from build123d import *

# Parameters (mm, degrees)
SKETCH1_R            = 11
SKETCH1_R_2          = 3
BOSS_EXTRUDE2_DEPTH  = 6
SKETCH3_R            = 10.5
CUT_EXTRUDE1_DEPTH   = 1
SKETCH4_R            = 3.55
BOSS_EXTRUDE5_DEPTH  = 1
SKETCH5_R            = 3.05
CUT_EXTRUDE2_DEPTH   = 17.673332001
BOSS_EXTRUDE6_START  = 2
SKETCH6_R            = 3.55
BOSS_EXTRUDE6_DEPTH  = 2
SKETCH7_R            = 3.05
CUT_EXTRUDE3_DEPTH   = 18.492855685
SKETCH9_R            = 11
BOSS_EXTRUDE9_DEPTH  = 6
SKETCH10_W           = 46.121208306
SKETCH10_H           = 4.65
BOSS_EXTRUDE10_DEPTH = 6


with BuildPart() as part:
    # Sketch1 → Boss-Extrude2 (new body)
    with BuildSketch(Plane.XY):
        Circle(SKETCH1_R)
        Circle(SKETCH1_R_2, mode=Mode.SUBTRACT)
    extrude(amount=BOSS_EXTRUDE2_DEPTH)

    # Sketch3 → Cut-Extrude1 (cut)
    with BuildSketch(Plane.XY.offset(6)):
        Circle(SKETCH3_R)
    extrude(amount=-CUT_EXTRUDE1_DEPTH, mode=Mode.SUBTRACT)

    # Sketch4 → Boss-Extrude5 (add)
    with BuildSketch(Plane.XY.offset(5)):
        Circle(SKETCH4_R)
    extrude(amount=BOSS_EXTRUDE5_DEPTH)

    # Sketch5 → Cut-Extrude2 (cut, through all)
    with BuildSketch(Plane.XY.offset(6)):
        Circle(SKETCH5_R)
    extrude(amount=-CUT_EXTRUDE2_DEPTH, mode=Mode.SUBTRACT)

    # Sketch6 → Boss-Extrude6 (add)
    with BuildSketch(Plane(origin=(0, 0, 0), x_dir=(-1, 0, 0), z_dir=(0, 0, -1)).offset(BOSS_EXTRUDE6_START)):
        with Locations(Location((0, 0, 0), (0, 0, 180))):
            Circle(SKETCH6_R)
    extrude(amount=-BOSS_EXTRUDE6_DEPTH)

    # Sketch7 → Cut-Extrude3 (cut, through all)
    with BuildSketch(Plane(origin=(0, 0, -2), x_dir=(-1, 0, 0), z_dir=(0, 0, -1))):
        with Locations(Location((0, 0, 0), (0, 0, 180))):
            Circle(SKETCH7_R)
    extrude(amount=-CUT_EXTRUDE3_DEPTH, mode=Mode.SUBTRACT)

    # Sketch9 → Boss-Extrude9 (add, through all)
    with BuildSketch(Plane.XY):
        with BuildLine():
            Line((-12.660604153, 0), (-12.660604153, -9.354915786))
            Line((-12.660604153, -9.354915786), (-23.060604153, -9.354915786))
            Line((-23.060604153, -9.354915786), (-23.060604153, -15.354915786))
            Line((-23.060604153, -15.354915786), (23.060604153, -15.354915786))
            Line((23.060604153, -15.354915786), (23.060604153, -9.354915786))
            Line((23.060604153, -9.354915786), (12.660604153, -9.354915786))
            Line((12.660604153, -9.354915786), (12.660604153, 0))
            ThreePointArc((12.660604153, 0), (0, 12.660604153), (-12.660604153, 0))
        make_face()
        Circle(SKETCH9_R, mode=Mode.SUBTRACT)
    extrude(amount=BOSS_EXTRUDE9_DEPTH)

    # Sketch10 → Boss-Extrude10 (add)
    with BuildSketch(Plane.XY):
        with Locations((0, -17.679915786)):
            Rectangle(SKETCH10_W, SKETCH10_H)
    extrude(amount=BOSS_EXTRUDE10_DEPTH)


solid = part.part
Design review of the part built by this model. Coordinates are the model's own, in mm. A direction names the side the tool comes from. Coordinates: 2 decimals unless noted, no trailing zeros. Order: outer loops, then holes, each group sorted by start corner. A loop starts at its lowest first (then second) coordinate and runs counter-clockwise, first axis right, second up. Notation, with made-up numbers: M 34,89.5 L 49,89.5 A21 ccw 49,120.5 Z; hole C 71,-35 d1. An arc over 180 degrees is marked long. Use a Markdown table: item, result.
(1) Add section A-A (x = 0). Give the boundary of the cut face in (y, z), then the cut area to 3 significant figures.
Worked answers:
| item | result |
|---|---|
| outline | M -20,0 L -3.55,0 L -3.55,-2 L -3.05,-2 L -3.05,6 L -3.55,6 L -3.55,5 L -10.5,5 L -10.5,6 L -20,6 Z; M 3.05,-2 L 3.55,-2 L 3.55,0 L 12.66,0 L 12.66,6 L 10.5,6 L 10.5,5 L 3.55,5 L 3.55,6 L 3.05,6 Z |
| area | 147 mm2 |
(2) Add section C-C (y = 1). Give the boundary of the cut face in (x, z), then the cut area to 3 significant figures.
Worked answers:
| item | result |
|---|---|
| outline | M -12.62,0 L -3.41,0 L -3.41,-2 L -2.88,-2 L -2.88,6 L -3.41,6 L -3.41,5 L -10.45,5 L -10.45,6 L -12.62,6 Z; M 2.88,-2 L 3.41,-2 L 3.41,0 L 12.62,0 L 12.62,6 L 10.45,6 L 10.45,5 L 3.41,5 L 3.41,6 L 2.88,6 Z |
| area | 105 mm2 |
(3) Wall thickness on probe 1 along Y at (x, z) = (0, 5.7); probe 2 along Y at (x, z) = (0, 3); probe 3 along Z at (x, y) = (-0.5, -6): over which ranges is each line inside the solid? List them lowest first.
Worked answers:
| item | result |
|---|---|
| probe 1 | y = -20 to -10.5, -3.55 to -3.05, 3.05 to 3.55, 10.5 to 12.66 |
| probe 2 | y = -20 to -3.05, 3.05 to 12.66 |
| probe 3 | z = 0 to 5 |
(4) For faces 1 (the cylindrical face through (-0.46, 3.52, 5.49)), 2 (the cylindrical face through (-0.46, -3.52, -1.01)), 3 (the flat face through (12.661, -5, 3)), 4 (the flat face through (-12.661, -5, 3)), list the 3-axis set-ups (+Z, -Z, +X, -X, +Y, -Y) from which the entire face can be reached by the end or side of a thin tool; tool diameter is ignored.
Worked answers:
| item | result |
|---|---|
| face 1 | +Z |
| face 2 | -Z |
| face 3 | +Z, -Z, +X, +Y |
| face 4 | +Z, -Z, -X, +Y |
(5) Add section D-D (y = -8). Give the boundary of the cut face in (x, z), then the cut area to 3 significant figures.
Worked answers:
| item | result |
|---|---|
| outline | M -12.66,0 L 12.66,0 L 12.66,6 L 6.8,6 L 6.8,5 L -6.8,5 L -6.8,6 L -12.66,6 Z |
| area | 138 mm2 |
(6) Draft analysis for pull direction X (two halves, no side actions). For faces 5 (the flat face through (5, 0, 5)), 6 (the flat face through (0, -7, 0)), 7 (the flat face through (-23.061, -15, 3)), state which applies: released by +X, released by -X, zero draft, split by the parting line, or undercut.
Worked answers:
| item | result |
|---|---|
| face 5 | undercut |
| face 6 | zero draft |
| face 7 | released by -X |
(7) For P1, Ø19, axis at x = 0, y = 0, coming from the -Z side; P2, Ø1, axis at x = -2.5, z = -1, coming from the -Y side; P3, Ø1.5, axis at x = 3, y = -10.5, coming from the -Z side; P4, Ø1.5, axis at x = 7, z = 0, coming from the +Y side, all flat-tipped, find the tip position at first contact; note any pin that passes through.
Worked answers:
| item | result |
|---|---|
| P1 | stops at z = -2 |
| P2 | stops at y = -2.93 |
| P3 | stops at z = 0 |
| P4 | stops at y = 11.01 |
(8) Add section B-B (z = 1). Give the boundary of the cut face in (x, y), then the cut area to 3 significant figures.
Worked answers:
| item | result |
|---|---|
| outline | M -23.06,-20 L 23.06,-20 L 23.06,-9.35 L 12.66,-9.35 L 12.66,0 A12.66 ccw -12.66,0 L -12.66,-9.35 L -23.06,-9.35 Z; hole C 0,0 d6.1 |
| area | 951 mm2 |
